For this review, use the dimensioned drawing (mm, ordinates from the lowest corner) and the shaded views. A direction names the side the tool comes from. Round coordinates to 2 decimals unless told otherwise and drop trailing zeros. Loops run counter-clockwise (first coordinate to the right, second up) from the corner with the lowest first, then second, coordinate; pieces in that order, holes last. Notation, with made-up numbers: M 81.25,-1 L 96.25,-1 A32 ccw 96.25,26 Z; hole C -23,81 d8. An arc over 180 degrees is marked long. One line per item, written item: value. Start each with the question number.
Item 1: We need section B-B (x = 30). Write out the cut boundary in (y, z).
Item 2: We need section C-C (y = 19). Write out the cut boundary in (x, z), then the cut area to 3 significant figures.
Item 3: We need section A-A (z = 23.5). Write out the cut boundary in (x, y), then the cut area to 3 significant figures.
Item 4: For line 1 along X through (y, z) = (29.5, 22); line 2 along Y through (x, z) = (108, 16); line 3 along Z through (x, y) = (177, 31), list the stretches that pass through material, from the lowest coordinate up.
Item 5: Mouldability with a two-part tool opening along Y and no side actions: class the marked faces 1, 2 and 3 as released by +Y, released by -Y, zero draft, split by the parting line, or undercut.
Item 6: Clearance check with flat-ended pins moving along their axes: pin 1 (4 mm diameter, centred on x = 148.5, y = 25, fed in from +Z); pin 2 (1.5 mm diameter, centred on x = 2, z = 34, fed in from -Y); pin 3 (1 mm diameter, centred on y = 44.5, z = 4.5, fed in from +X). State where each tip first meets the part, or that it passes through.
Item 7: For the marked faces 4 and 5, list the 3-axis set-ups (+Z, -Z, +X, -X, +Y, -Y) from which the entire face can be reached by the end or side of a thin tool; tool diameter is ignored.
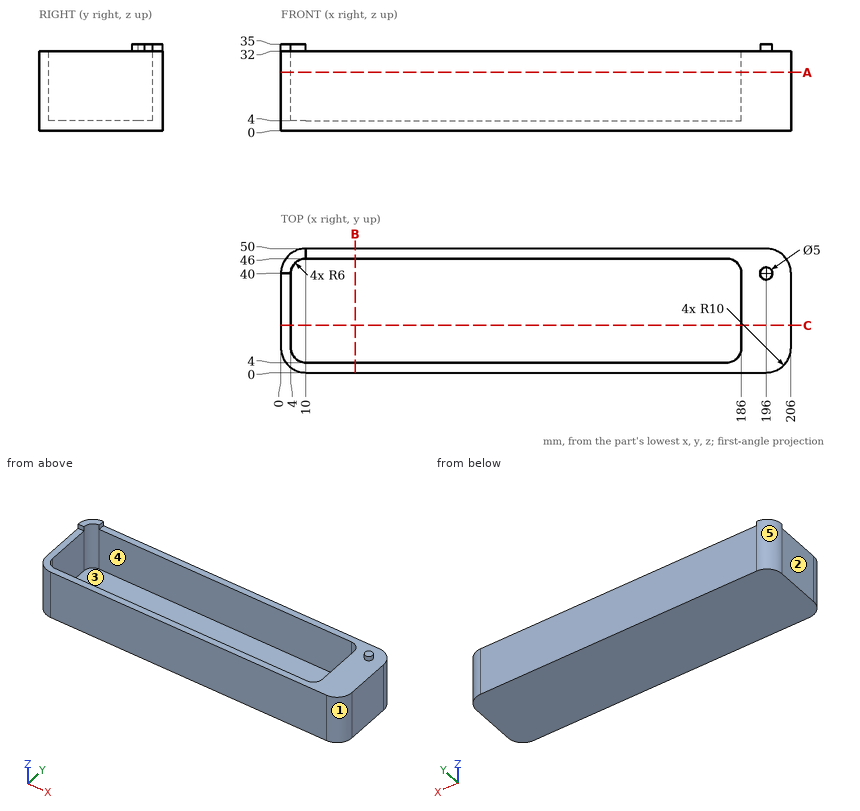
A:
1. outline: M 0,0 L 50,0 L 50,32 L 46,32 L 46,4 L 4,4 L 4,32 L 0,32 Z
2. outline: M 0,0 L 206,0 L 206,32 L 186,32 L 186,4 L 4,4 L 4,32 L 0,32 Z
2. area: 1,500 mm2
3. outline: M 0,10 A10 ccw 10,0 L 196,0 A10 ccw 206,10 L 206,40 A10 ccw 196,50 L 10,50 A10 ccw 0,40 Z; hole M 4,10 A6 ccw 10,4 L 180,4 A6 ccw 186,10 L 186,40 A6 ccw 180,46 L 10,46 A6 ccw 4,40 Z
3. area: 2,600 mm2
4. line 1: 0 to 4, 186 to 206
4. line 2: 0 to 4, 46 to 50
4. line 3: 0 to 4
5. face 1: released by -Y
5. face 2: zero draft
5. face 3: undercut
6. pin 1: z = 4
6. pin 2: y = 40
6. pin 3: x = 205.17
7. face 4: +Z
7. face 5: +Z, -Z, -X, +Y
